Input: part model. Units: mm. Frame: model coordinates. Coordinates: 2 decimals unless noted, no trailing zeros. Write each loop counter-clockwise with the first axis right and the second up, starting at its lowest first coordinate (ties: lowest second). Pieces come first, ordered by that corner, then holes. Notation, with made-up numbers: (53.25, 33) -> (58.25, 33) arc R16 cw to (58.25, 41) -> close; hole circle Ø7 at (-12.5, 49.25). An arc over 180 degrees is marked (long way). Use one line per item in the form item = value. Start each with the question number.
(1) Ray query, line 1 along X through (y, z) = (2.1, -4.75); line 2 along X through (y, z) = (2.1, -11.25); line 3 along Z through (x, y) = (10, 0.65). Return the intervals inside material, ascending.
(2) Cut plane B-B on x = 9.5. Return the cut outline in (y, z).
(3) Cut plane A-A on y = 1.95. Return the cut outline in (x, z), plus the area to 3 significant figures.
```python
from build123d import *

# Parameters (mm, degrees)
SKETCH2_W            = 128.35
SKETCH2_H            = 20
BOSS_EXTRUDE1_DEPTH  = 5
M3_CLEARANCE_HOLE1_D = 3.6
M3_CLEARANCE_HOLE2_D = 3.6


with BuildPart() as part:
    # Sketch2 → Boss-Extrude1 (new body)
    with BuildSketch(Plane(origin=(0, 0, 0), x_dir=(1, 0, 0), z_dir=(0, 1, 0))):
        with Locations((24.337601626, 10.975609756)):
            Rectangle(SKETCH2_W, SKETCH2_H)
    extrude(amount=BOSS_EXTRUDE1_DEPTH)

    # M3 Clearance Hole1 (through all)
    with Locations(Plane(origin=(0, 5, 0), x_dir=(1, 0, 0), z_dir=(0, 1, 0))):
        with Locations((-36.662398374, 16.975609756), (-36.662398374, 4.975609756), (85.337601626, 16.975609756), (85.337601626, 4.975609756)):
            Hole(M3_CLEARANCE_HOLE1_D / 2)

    # M3 Clearance Hole2 (through all)
    with Locations(Plane(origin=(0, 5, 0), x_dir=(1, 0, 0), z_dir=(0, 1, 0))):
        with Locations((9.337601626, 10.975609756), (39.337601626, 10.975609756)):
            Hole(M3_CLEARANCE_HOLE2_D / 2)


solid = part.part
```
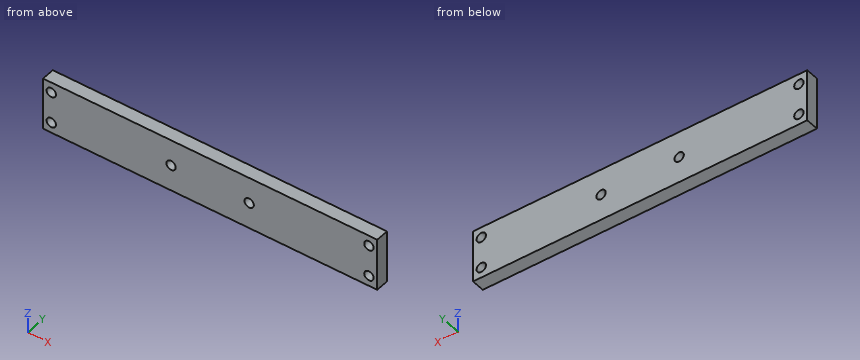
Values:
q1.line_1 = -39.84 to -38.45, -34.88 to 83.55, 87.12 to 88.51
q1.line_2 = -39.84 to 7.56, 11.12 to 37.56, 41.12 to 88.51
q1.line_3 = -20.98 to -12.65, -9.3 to -0.98
q2.outline = (0, -20.98) -> (5, -20.98) -> (5, -12.77) -> (0, -12.77) -> close; (0, -9.18) -> (5, -9.18) -> (5, -0.98) -> (0, -0.98) -> close
q3.outline = (-39.84, -20.98) -> (88.51, -20.98) -> (88.51, -0.98) -> (-39.84, -0.98) -> close; hole circle Ø3.6 at (-36.66, -16.98); hole circle Ø3.6 at (-36.66, -4.98); hole circle Ø3.6 at (9.34, -10.98); hole circle Ø3.6 at (39.34, -10.98); hole circle Ø3.6 at (85.34, -16.98); hole circle Ø3.6 at (85.34, -4.98)
q3.area = 2,510 mm2
